Here's how the part is built. I have some questions about the finished solid (model axes, mm). A direction names the side the tool comes from. Round coordinates to 2 decimals unless told otherwise and drop trailing zeros. Order: outer loops, then holes, each group sorted by start corner. A loop starts at its lowest first (then second) coordinate and runs counter-clockwise, first axis right, second up. Notation, with made-up numbers: (77.5, 10.25) -> (107.5, 10.25) arc R12 cw to (107.5, 27.25) -> close; hole circle Ø3 at (57, 82.25). An arc over 180 degrees is marked (long way). Answer in a Markdown table with one row per item.
```python
from build123d import *

# Parameters (mm, degrees)
SKETCH1_R               = 13.5
BOSS_EXTRUDE1_DEPTH     = 22.5
SKETCH2_W               = 60.5
SKETCH2_H               = 60.5
CUT_EXTRUDE1_DEPTH      = 28.5
SKETCH3_R               = 25.25
CUT_EXTRUDE2_DEPTH      = 3
SKETCH4_R               = 2.3
CUT_EXTRUDE3_DEPTH      = 29.5
CUT_EXTRUDE3_DEPTH_BACK = 17.5
CHAMFER1_SIZE           = 3
SKETCH5_R               = 3.05
CUT_EXTRUDE4_DEPTH      = 80.75
SKETCH6_R               = 5.5
CUT_EXTRUDE5_DEPTH      = 37.25
FILLET1_R               = 3
FILLET2_R               = 6
FILLET3_R               = 2
CHAMFER2_SIZE           = 3
CUT_EXTRUDE6_DEPTH      = 1
CUT_EXTRUDE6_DEPTH_BACK = 81


with BuildPart() as part:
    # Sketch1 → Boss-Extrude1 (new body, symmetric)
    with BuildSketch(Plane.XY):
        Polygon((40, -79.75), (25.85, -79.75), (25.85, -55.45), (-25.85, -55.45), (-25.85, -79.75), (-40, -79.75), (-40, 30.25), (40, 30.25), align=None)
        Circle(SKETCH1_R, mode=Mode.SUBTRACT)
    extrude(amount=BOSS_EXTRUDE1_DEPTH, both=True)

    # Sketch2 → Cut-Extrude1 (cut)
    with BuildSketch(Plane.XY.offset(22.5)):
        Rectangle(SKETCH2_W, SKETCH2_H)
    extrude(amount=-CUT_EXTRUDE1_DEPTH, mode=Mode.SUBTRACT)

    # Sketch3 → Cut-Extrude2 (cut)
    with BuildSketch(Plane.XY.offset(-6)):
        Circle(SKETCH3_R)
    extrude(amount=-CUT_EXTRUDE2_DEPTH, mode=Mode.SUBTRACT)

    # Sketch4 → Cut-Extrude3 (cut, two sides)
    with BuildSketch(Plane.XY.offset(-6)) as cut_extrude3_sk:
        with Locations((-25, 25)):
            Circle(SKETCH4_R)
        with Locations((25, 25)):
            Circle(SKETCH4_R)
        with Locations((25, -25)):
            Circle(SKETCH4_R)
        with Locations((-25, -25)):
            Circle(SKETCH4_R)
    extrude(amount=CUT_EXTRUDE3_DEPTH, mode=Mode.SUBTRACT)
    extrude(cut_extrude3_sk.sketch, amount=-CUT_EXTRUDE3_DEPTH_BACK, mode=Mode.SUBTRACT)

    # Chamfer1
    chamfer1_edges = [part.edges().sort_by_distance(p)[0] for p in [
        (-13.5, 0, -22.5),
    ]]
    chamfer(chamfer1_edges, length=CHAMFER1_SIZE)

    # Sketch5 → Cut-Extrude4 (cut, through all)
    with BuildSketch(Plane(origin=(0, 0, 0), x_dir=(1, 0, 0), z_dir=(0, 1, 0))):
        with Locations((0, 8.5)):
            Circle(SKETCH5_R)
        with Locations((0, -14)):
            Circle(SKETCH5_R)
    extrude(amount=-CUT_EXTRUDE4_DEPTH, mode=Mode.SUBTRACT)

    # Sketch6 → Cut-Extrude5 (cut)
    with BuildSketch(Plane(origin=(0, 0, 0), x_dir=(1, 0, 0), z_dir=(0, 1, 0))):
        with Locations((0, -14)):
            Circle(SKETCH6_R)
        with Locations((0, 8.5)):
            Circle(SKETCH6_R)
    extrude(amount=-CUT_EXTRUDE5_DEPTH, mode=Mode.SUBTRACT)

    # Fillet1
    fillet1_edges = [part.edges().sort_by_distance(p)[0] for p in [
        (-30.25, -30.25, 8.25),
        (30.25, -30.25, 8.25),
    ]]
    fillet(fillet1_edges, radius=FILLET1_R)

    # Fillet2
    fillet2_edges = [part.edges().sort_by_distance(p)[0] for p in [
        (25.85, -55.45, 0),
        (-25.85, -55.45, 0),
    ]]
    fillet(fillet2_edges, radius=FILLET2_R)

    # Fillet3
    fillet3_edges = [part.edges().sort_by_distance(p)[0] for p in [
        (5.477225575, -18.493872805, -9),
        (-5.477225575, -18.493872805, -9),
        (4.898979486, -27.510096891, -6),
        (-4.898979486, -27.510096891, -6),
    ]]
    fillet(fillet3_edges, radius=FILLET3_R)

    # Chamfer2
    chamfer2_edges = [part.edges().sort_by_distance(p)[0] for p in [
        (-40, 30.25, 0),
        (40, 30.25, 0),
        (40, -79.75, 0),
        (-40, -79.75, 0),
    ]]
    chamfer(chamfer2_edges, length=CHAMFER2_SIZE)

    # Sketch7 → Cut-Extrude6 (cut, two sides)
    with BuildSketch(Plane(origin=(40, 0, 0), x_dir=(0, 0, -1), z_dir=(1, 0, 0))) as cut_extrude6_sk:
        Polygon((-8.512452887, 30.25), (-22.5, 3.260250001), (-22.5, 30.25), align=None)
    extrude(amount=CUT_EXTRUDE6_DEPTH, mode=Mode.SUBTRACT)
    extrude(cut_extrude6_sk.sketch, amount=-CUT_EXTRUDE6_DEPTH_BACK, mode=Mode.SUBTRACT)


solid = part.part
```
1. Please list where these lines run through material, in increasing order: line 1 along Z through (x, y) = (0, -50.5); line 2 along X through (y, z) = (0, -9.15); line 3 along X through (y, z) = (-33, 14.5).
Numbers:
| item | result |
|---|---|
| line 1 | z = -22.5 to -11.55, -5.45 to 10.95, 17.05 to 22.5 |
| line 2 | x = -40 to -13.5, 13.5 to 40 |
| line 3 | x = -40 to -5.48, 5.48 to 40 |
2. Suppose I cut it at B-B on x = 0. Write out the boundary of the cut face in (y, z).
Numbers:
| item | result |
|---|---|
| outline | (-55.45, -22.5) -> (-16.5, -22.5) -> (-13.5, -19.5) -> (-13.5, -14) -> (-37.25, -14) -> (-37.25, -11.55) -> (-55.45, -11.55) -> close; (-55.45, -5.45) -> (-37.25, -5.45) -> (-37.25, -3) -> (-30.25, -3) -> (-30.25, 8.5) -> (-37.25, 8.5) -> (-37.25, 10.95) -> (-55.45, 10.95) -> close; (-55.45, 17.05) -> (-37.25, 17.05) -> (-37.25, 19.5) -> (-30.25, 19.5) -> (-30.25, 22.5) -> (-55.45, 22.5) -> close; (13.5, -19.5) -> (16.5, -22.5) -> (30.25, -22.5) -> (30.25, -6) -> (25.25, -6) -> (25.25, -9) -> (13.5, -9) -> close |
3. For pin 1 Ø10 at (x, z) = (-21, -6.5) entering from -Y; pin 2 Ø14.5 at (x, z) = (0, 14) entering from +Y; pin 3 Ø5.5 at (x, z) = (2, 14) entering from +Y; pin 4 Ø5.5 at (x, y) = (25, 25) entering from +Z, each with a flat end and sliding along its axis, tell me the tip position at first contact or that it passes through.
Numbers:
| item | result |
|---|---|
| pin 1 | stops at y = -79.75 |
| pin 2 | stops at y = -30.25 |
| pin 3 | stops at y = -37.25 |
| pin 4 | stops at z = -6 |
4. For faces 4 (the face through (-0.716, -27.438, -13.953)), 5 (the face through (0, 27, -6)), 6 (the face through (1.64, -46.22, -11.07)), 7 (the face through (0, -55.45, 0)), which set-ups out of +Z, -Z, +X, -X, +Y, -Y let a thin tool reach every point of the face, with its end or its side?
Numbers:
| item | result |
|---|---|
| face 4 | none |
| face 5 | +Z, +Y |
| face 6 | -Y |
| face 7 | +Z, -Z, -Y |
5. Suppose I cut it at D-D on y = -45.5. Write out the boundary of the cut face in (x, z), then the cut area to 3 significant figures.
Numbers:
| item | result |
|---|---|
| outline | (-40, -22.5) -> (40, -22.5) -> (40, 22.5) -> (-40, 22.5) -> close; hole circle Ø6.1 at (0, -8.5); hole circle Ø6.1 at (0, 14) |
| area | 3,540 mm2 |
6. Suppose I cut it at C-C on z = 6. Write out the boundary of the cut face in (x, y), then the cut area to 3 significant figures.
Numbers:
| item | result |
|---|---|
| outline | (-40, -76.75) -> (-37, -79.75) -> (-25.85, -79.75) -> (-25.85, -61.45) arc R6 cw to (-19.85, -55.45) -> (19.85, -55.45) arc R6 cw to (25.85, -61.45) -> (25.85, -79.75) -> (37, -79.75) -> (40, -76.75) -> (40, 27.25) -> (37, 30.25) -> (30.25, 30.25) -> (30.25, -27.25) arc R3 cw to (27.25, -30.25) -> (-27.25, -30.25) arc R3 cw to (-30.25, -27.25) -> (-30.25, 30.25) -> (-37, 30.25) -> (-40, 27.25) -> close |
| area | 3,880 mm2 |
7. Suppose I cut it at A-A on y = 0. Write out the boundary of the cut face in (x, z).
Numbers:
| item | result |
|---|---|
| outline | (-40, -22.5) -> (-16.5, -22.5) -> (-13.5, -19.5) -> (-13.5, -9) -> (-25.25, -9) -> (-25.25, -6) -> (-30.25, -6) -> (-30.25, 22.5) -> (-40, 22.5) -> close; (13.5, -19.5) -> (16.5, -22.5) -> (40, -22.5) -> (40, 22.5) -> (30.25, 22.5) -> (30.25, -6) -> (25.25, -6) -> (25.25, -9) -> (13.5, -9) -> close |
8. We'd pull the mould along Y, two halves only. Please class faces 1 (the face through (-38.52, -78.23, -0.31)), 2 (the face through (1, -47, 22.5)), 3 (the face through (26.06, 22.96, -14.13)): released by +Y, released by -Y, zero draft, split by the parting line, or undercut.
Numbers:
| item | result |
|---|---|
| face 1 | released by -Y |
| face 2 | zero draft |
| face 3 | undercut |
